Can you work these out from the drawing? Everything is in mm from the part's minimum corner. A direction names the side the tool comes from. Coordinates: 2 decimals unless noted, no trailing zeros. Loops run counter-clockwise (first coordinate to the right, second up) from the corner with the lowest first, then second, coordinate; pieces in that order, holes last. Notation, with made-up numbers: (13, -37.75) -> (50, -37.75) arc R29 ccw to (50, -9.75) -> close; hole circle Ø4 at (-8.5, 5). An arc over 180 degrees is marked (long way). Put each result on its own line as item: value. Start each with the question number.
Item 1: For the marked faces 1, 2 and 3, which set-ups out of +Z, -Z, +X, -X, +Y, -Y let a thin tool reach every point of the face, with its end or its side?
Item 2: If we section it at D-D on z = 45: Please give me the cut outline in (x, y), plus the area to 3 significant figures.
Item 3: We'd pull the mould along Z, two halves only. Please class the marked faces 4, 5, 6 and 7: pulls with the +Z half, pulls with the -Z half, needs draft (parallel to the pull), parting line crosses it, or undercut.
Item 4: Will these pins go through, and if not, where does the flat tip stop? P1, Ø8, axis at y = 10, z = 27, coming from the +X side (1 decimal); P2, Ø4, axis at y = 13, z = 41.5, coming from the +X side (1 decimal); P3, Ø1.5, axis at x = 37.5, y = 9.5, coming from the +Z side (1 decimal).
Item 5: Please list where these lines run through material, in increasing order: L1, parallel to Y at x = 31.5, z = 46; L2, parallel to X at y = 19, z = 24; L3, parallel to Z at x = 26.5, y = 26. Write a range as from..to.
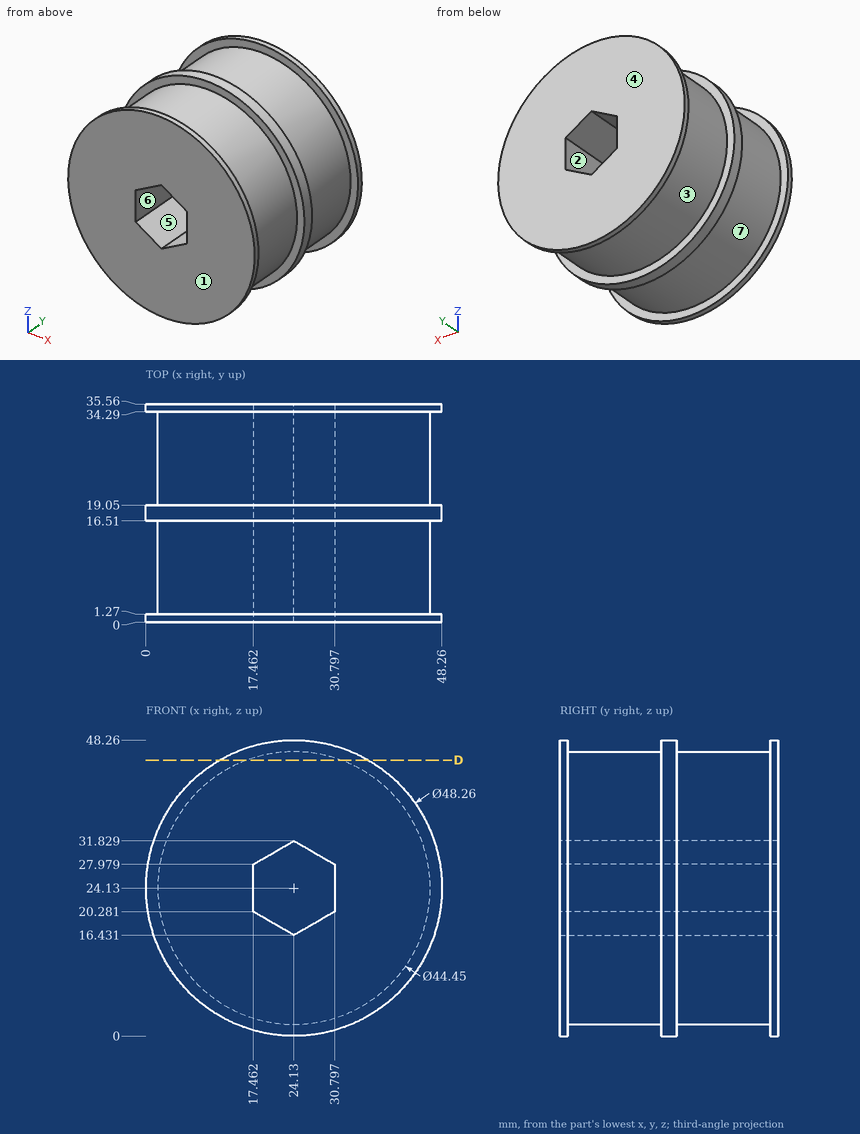
Solutions:
1. face 1: +Z, -Z, +X, -X, -Y
1. face 2: +Y, -Y
1. face 3: none
2. outline: (12.02, 0) -> (36.24, 0) -> (36.24, 1.27) -> (31.77, 1.27) -> (31.77, 16.51) -> (36.24, 16.51) -> (36.24, 19.05) -> (31.77, 19.05) -> (31.77, 34.29) -> (36.24, 34.29) -> (36.24, 35.56) -> (12.02, 35.56) -> (12.02, 34.29) -> (16.49, 34.29) -> (16.49, 19.05) -> (12.02, 19.05) -> (12.02, 16.51) -> (16.49, 16.51) -> (16.49, 1.27) -> (12.02, 1.27) -> close
2. area: 589 mm^2
3. face 4: needs draft
3. face 5: undercut
3. face 6: undercut
3. face 7: parting line crosses it
4. P1: x = 46.4
4. P2: x = 40.2
4. P3: z = 42.4
5. L1: 0..1.27, 16.51..19.05, 34.29..35.56
5. L2: 0..17.46, 30.8..48.26
5. L3: 2.03..17.8, 30.46..46.23
